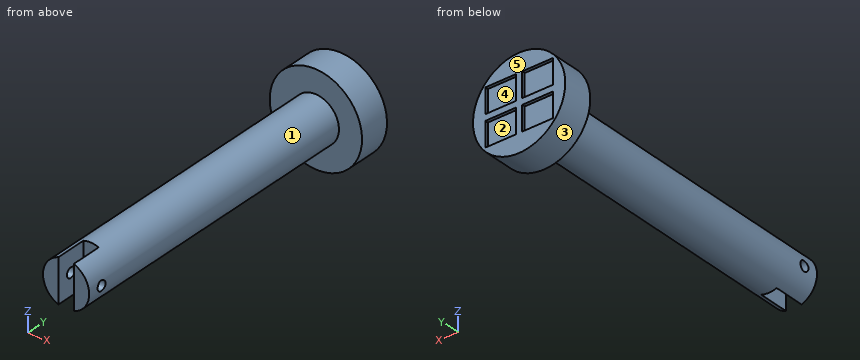
from build123d import *

# Parameters (mm, degrees)
SKETCH_1_R               = 7.5
EXTRUDE_1_DEPTH          = 100
SKETCH_2_R               = 15
EXTRUDE_2_DEPTH          = 10
CUT_EXTRUDE_1_DEPTH      = 113.026782512
CUT_EXTRUDE_1_DEPTH_BACK = 113.026782512
SKETCH_3_W               = 5
SKETCH_3_H               = 10
CUT_EXTRUDE_2_DEPTH      = 113.026782512
CUT_EXTRUDE_2_DEPTH_BACK = 113.026782512
SKETCH_4_R               = 1.6
SKETCH_5_W               = 10
SKETCH_5_H               = 8
CUT_EXTRUDE_3_DEPTH      = 1


with BuildPart() as part:
    # ｽｹｯﾁ1 → ﾎﾞｽ - 押し出し1 (new body)
    with BuildSketch(Plane(origin=(0, 0, 0), x_dir=(1, 0, 0), z_dir=(0, 1, 0))):
        with Locations(Location((0, 0, 0), (0, 0, 270))):
            Circle(SKETCH_1_R)
    extrude(amount=EXTRUDE_1_DEPTH)

    # ｽｹｯﾁ2 → ﾎﾞｽ - 押し出し2 (add)
    with BuildSketch(Plane(origin=(0, 100, 0), x_dir=(1, 0, 0), z_dir=(0, 1, 0))):
        with Locations(Location((0, 0, 0), (0, 0, 270))):
            Circle(SKETCH_2_R)
    extrude(amount=EXTRUDE_2_DEPTH)

    # ｽｹｯﾁ3 → ｶｯﾄ - 押し出し1 (cut, two sides: drawn at the far end of the back side and taken through both)
    with BuildSketch(Plane.XY.offset(-CUT_EXTRUDE_1_DEPTH_BACK)):
        with Locations((0, 5)):
            Rectangle(SKETCH_3_W, SKETCH_3_H)
    extrude(amount=CUT_EXTRUDE_1_DEPTH + CUT_EXTRUDE_1_DEPTH_BACK, mode=Mode.SUBTRACT)

    # ｽｹｯﾁ4 → ｶｯﾄ - 押し出し2 (cut, two sides: drawn at the far end of the back side and taken through both)
    with BuildSketch(Plane(origin=(0, 0, 0), x_dir=(0, 0, -1), z_dir=(1, 0, 0)).offset(-CUT_EXTRUDE_2_DEPTH_BACK)):
        with Locations((0, 5)):
            Circle(SKETCH_4_R)
    extrude(amount=CUT_EXTRUDE_2_DEPTH + CUT_EXTRUDE_2_DEPTH_BACK, mode=Mode.SUBTRACT)

    # ｽｹｯﾁ5 → ｶｯﾄ - 押し出し3 (cut)
    with BuildSketch(Plane(origin=(0, 110, 0), x_dir=(1, 0, 0), z_dir=(0, 1, 0))):
        with Locations((-6, 5)):
            Rectangle(SKETCH_5_W, SKETCH_5_H)
        with Locations((6, 5)):
            Rectangle(SKETCH_5_W, SKETCH_5_H)
        with Locations((6, -5)):
            Rectangle(SKETCH_5_W, SKETCH_5_H)
        with Locations((-6, -5)):
            Rectangle(SKETCH_5_W, SKETCH_5_H)
    extrude(amount=-CUT_EXTRUDE_3_DEPTH, mode=Mode.SUBTRACT)


solid = part.part
Geometry check sheet. Reference: the model listing, model coordinates, mm. Face numbers are marked on the shaded views. A direction names the side the tool comes from. Round coordinates to 2 decimals unless told otherwise and drop trailing zeros. Order: outer loops, then holes, each group sorted by start corner. A loop starts at its lowest first (then second) coordinate and runs counter-clockwise, first axis right, second up. Notation, with made-up numbers: (25.25, 48) - (30.25, 48) arc R27 ccw to (30.25, 87) - close; hole circle Ø6 at (56, 73.5). An arc over 180 degrees is marked (long way). One line per question, with ' | ' between items. Start each with the question number.
(1) Thickness scan on L1, parallel to Y at x = -5.85, z = 0; L2, parallel to Y at x = -5.5, z = -9.75; L3, parallel to X at y = 81.5, z = 0.25. Record the ranges inside material, lowest first. Write a range as [from, to].
(2) Depth check by flat-ended pin: pin 1 Ø0.8 at (y, z) = (109.5, 6.5) entering from +X; pin 2 Ø1.1 at (y, z) = (109.5, 4) entering from -X; pin 3 Ø2.5 at (x, z) = (-8, 6) entering from +Y; pin 4 Ø2 at (x, z) = (3.5, -7) entering from -Y. Enter the tip coordinate at first touch or a pass-through.
(3) Sectioned sample at C-C on y = 9. Record the cut outline in (x, z).
(4) Release check for a two-part mould opening along Z. For the marked faces 3, 4 and 5 record: released by +Z, released by -Z, zero draft, split by the parting line, or undercut.
(5) Sectioned sample at D-D on y = 38.5. Record the cut outline in (x, z).
(6) Access from +Z, -Z, +X, -X, +Y, -Y to the whole of each face (thin tool, end or side, straight path). Record for the marked faces 1 and 2.
(7) Sectioned sample at A-A on z = 0. Record the cut outline in (x, y).
(8) Sectioned sample at B-B on x = 0. Record the cut outline in (y, z).
Conclusion:
1) L1: y = [0, 3.4], [6.6, 110] | L2: y = [100, 110] | L3: x = [-7.5, 7.5]
2) pin 1: stops at x = 13.7 | pin 2: stops at x = -14.6 | pin 3: stops at y = 109 | pin 4: stops at y = 0
3) outline: (-2.5, -7.07) - (-2.5, 7.07) arc R7.5 ccw to start; (2.5, -7.07) arc R7.5 ccw to (2.5, 7.07) - close
4) face 3: split by the parting line | face 4: undercut | face 5: zero draft
5) outline: circle Ø15 at (0, 0)
6) face 1: -Y | face 2: +Y
7) outline: (-15, 100) - (-7.5, 100) - (-7.5, 6.6) - (-2.5, 6.6) - (-2.5, 10) - (2.5, 10) - (2.5, 6.6) - (7.5, 6.6) - (7.5, 100) - (15, 100) - (15, 110) - (-15, 110) - close; (-7.5, 0) - (-2.5, 0) - (-2.5, 3.4) - (-7.5, 3.4) - close; (2.5, 0) - (7.5, 0) - (7.5, 3.4) - (2.5, 3.4) - close
8) outline: (10, -7.5) - (100, -7.5) - (100, -15) - (110, -15) - (110, 15) - (100, 15) - (100, 7.5) - (10, 7.5) - close
